from build123d import *

# Parameters (mm, degrees)
F0_W     = 1016
F0_H     = 406.4
F0_W_2   = 38.1
F0_H_2   = 330.2
F1_DEPTH = 38.1


with BuildPart() as f1:
    # F0 (on Top) → F1 (new body)
    with BuildSketch(Plane.XY):
        Rectangle(F0_W, F0_H)
        Polygon((469.9, 165.1), (469.9, -165.1), (19.05, -165.1), (-19.05, -165.1), (-469.9, -165.1), (-469.9, 165.1), (-19.05, 165.1), (19.05, 165.1), align=None, mode=Mode.SUBTRACT)
        Rectangle(F0_W_2, F0_H_2)
    extrude(amount=F1_DEPTH)


solid = f1.part
Model file for the job. Use its own axes, mm. A direction names the side the tool comes from. Give positions to 0.01 mm unless a question says otherwise; leave off trailing zeros. Order: outer loops, then holes, each group sorted by start corner. A loop starts at its lowest first (then second) coordinate and runs counter-clockwise, first axis right, second up. Notation, with made-up numbers: (60, 79.25) - (92, 79.25) arc R15 cw to (92, 100.25) - close; hole circle Ø1 at (11, 38.25). An arc over 180 degrees is marked (long way). One line per item, written item: value.
Item 1: Wall check: line 1 (X direction, y = -51, z = 36.5); line 2 (Y direction, x = 445, z = 28). Give the ranges that are in metal, low to high.
Response values:
line 1: -508 to -469.9, -19.05 to 19.05, 469.9 to 508
line 2: -203.2 to -165.1, 165.1 to 203.2
Item 2: Tool access for faces 1 (the flat face through (241, 165.1, 19)), 2 (the flat face through (-508, -3, 19)): list every direction of +Z, -Z, +X, -X, +Y, -Y with a clear straight run to the whole face (end or side of a thin tool).
Response values:
face 1: +Z, -Z
face 2: +Z, -Z, -X, +Y, -Y
Item 3: Slice it at C-C (x = 297.5). List the corners of the cut face in (y, z).
Response values:
outline: (-203.2, 0) - (-165.1, 0) - (-165.1, 38.1) - (-203.2, 38.1) - close; (165.1, 0) - (203.2, 0) - (203.2, 38.1) - (165.1, 38.1) - close
Item 4: Slice it at B-B (z = 7). List the corners of the cut face in (x, y).
Response values:
outline: (-508, -203.2) - (508, -203.2) - (508, 203.2) - (-508, 203.2) - close; hole (-469.9, -165.1) - (-19.05, -165.1) - (-19.05, 165.1) - (-469.9, 165.1) - close; hole (19.05, -165.1) - (469.9, -165.1) - (469.9, 165.1) - (19.05, 165.1) - close
Item 5: Slice it at A-A (y = 95). List the corners of the cut face in (x, z), then the cut area to 3 significant figures.
Response values:
outline: (-508, 0) - (-469.9, 0) - (-469.9, 38.1) - (-508, 38.1) - close; (-19.05, 0) - (19.05, 0) - (19.05, 38.1) - (-19.05, 38.1) - close; (469.9, 0) - (508, 0) - (508, 38.1) - (469.9, 38.1) - close
area: 4,350 mm2
